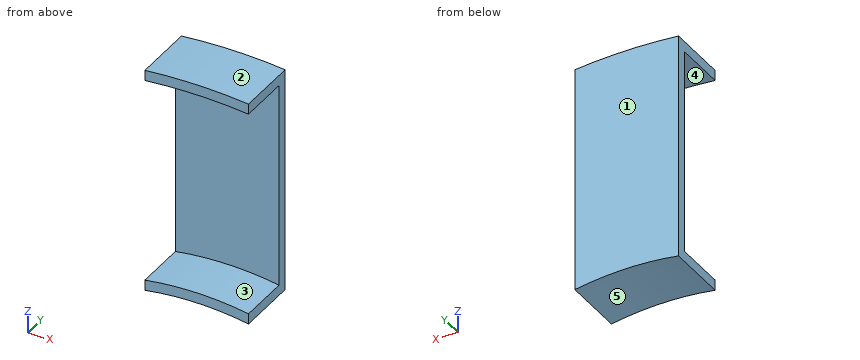
from build123d import *

# Parameters (mm, degrees)
BOSS_EXTRUDE1_DEPTH = 5
SHELL2_T            = 1


with BuildPart() as part:
    # Sketch1 → Boss-Extrude1 (new body)
    with BuildSketch(Plane(origin=(0, 0, 0), x_dir=(1, 0, 0), z_dir=(0, 1, 0))):
        with BuildLine():
            ThreePointArc((-5, -49.787563146), (0, -50.038), (5, -49.787563146))
            Line((5, -49.787563146), (5, -29.873965426))
            ThreePointArc((5, -29.873965426), (0, -30.2895), (-5, -29.873965426))
            Line((-5, -29.873965426), (-5, -49.787563146))
        make_face()
    extrude(amount=BOSS_EXTRUDE1_DEPTH)

    # Shell2
    shell2_openings = [part.faces().sort_by_distance(p)[0] for p in [
        (5, 2.5, 39.830764286),
        (-5, 2.5, 39.830764286),
        (0, 0, 40.052741683),
    ]]
    offset(amount=SHELL2_T, openings=shell2_openings, kind=Kind.INTERSECTION)


solid = part.part
Model file for the job. Use its own axes, mm. Face numbers are marked on the shaded views. A direction names the side the tool comes from. Give positions to 0.01 mm unless a question says otherwise; leave off trailing zeros. Loops run counter-clockwise (first coordinate to the right, second up) from the corner with the lowest first, then second, coordinate; pieces in that order, holes last.
1) Pull direction Z, two halves, no side cores. Call the marked faces 1, 2 and 3: +Z half, -Z half, draft (parallel to the pull), parting line (faces both ways), or undercut.
2) Flat gauge pins, fed straight in: pin 1 Ø4 at (x, z) = (0, 48) entering from -Y; pin 2 Ø1.5 at (x, y) = (-3.5, 4.5) entering from -Z. Where does each tip first touch, or does it go through?
3) Wall check: line 1 (Z direction, x = -0.25, y = 4.55); line 2 (Y direction, x = -4, z = 49.25); line 3 (Z direction, x = 3.75, y = 0.55). Give the ranges that are in metal, low to high.
4) Saw through at D-D (x = 0.5). Write the cut outline in (y, z), plus the area to 3 significant figures.
5) Saw through at C-C (z = 40.75). Write the cut outline in (x, y).
6) Saw through at B-B (x = 4). Write the cut outline in (y, z).
7) Tool access for the marked faces 4 and 5: list every direction of +Z, -Z, +X, -X, +Y, -Y with a clear straight run to the whole face (end or side of a thin tool).
8) Saw through at A-A (y = 3.9). Write the cut outline in (x, z).
Answer block:
1. face 1: draft
1. face 2: +Z half
1. face 3: undercut
2. pin 1: stops at y = 5
2. pin 2: stops at z = 28.98
3. line 1: z = 29.29 to 30.29, 50.04 to 51.04
3. line 2: y = 5 to 6
3. line 3: z = 29.05 to 30.06, 49.9 to 50.9
4. outline: (0, 29.29) - (6, 29.29) - (6, 51.04) - (0, 51.04) - (0, 50.04) - (5, 50.04) - (5, 30.29) - (0, 30.29) - close
4. area: 31.8 mm2
5. outline: (-5, 5) - (5, 5) - (5, 6) - (-5, 6) - close
6. outline: (0, 29.02) - (6, 29.02) - (6, 50.88) - (0, 50.88) - (0, 49.88) - (5, 49.88) - (5, 30.02) - (0, 30.02) - close
7. face 4: -Y
7. face 5: -Z, +Y, -Y
8. outline: (-5, 28.86) arc R29.29 cw to (5, 28.86) - (5, 29.87) arc R30.29 ccw to (-5, 29.87) - close; (-5, 49.79) arc R50.04 cw to (5, 49.79) - (5, 50.79) arc R51.04 ccw to (-5, 50.79) - close
